from build123d import *

# Parameters (mm, degrees)
PAD001_DEPTH    = 28.5
SKETCH002_R     = 14.25
POCKET_DEPTH    = 18.5
SKETCH003_R     = 1.375
POCKET001_DEPTH = 10
CHAMFER_SIZE    = 1
SKETCH004_W     = 10.5
SKETCH004_H     = 4
POCKET002_DEPTH = 10
SKETCH008_R     = 3
POCKET004_DEPTH = 5
SKETCH009_R     = 1.75
POCKET005_DEPTH = 5
CHAMFER004_SIZE = 0.5
SKETCH012_R     = 1.375
POCKET008_DEPTH = 8
SKETCH013_R     = 1.375
POCKET009_DEPTH = 8
CHAMFER005_SIZE = 1


with BuildPart() as motorbracketgroovemirrored001:
    # Sketch001 → Pad001 (new body)
    with BuildSketch(Plane.YZ):
        with BuildLine():
            ThreePointArc((2.474858, 19.974889), (-1.339402, 20.733574), (-3.5, 17.5))
            Line((-3.5, 17.5), (-3.5, -17.5))
            ThreePointArc((-3.5, -17.5), (-1.339402, -20.733574), (2.474858, -19.974889))
            Line((4.5, -17.949747), (2.474858, -19.974889))
            Line((4.5, 17.949747), (4.5, -17.949747))
            Line((4.5, 17.949747), (2.474858, 19.974889))
        make_face()
    extrude(amount=PAD001_DEPTH)

    # Sketch002 → Pocket (cut)
    with BuildSketch(Plane.YZ.offset(28.5)):
        Circle(SKETCH002_R)
    extrude(amount=-POCKET_DEPTH, mode=Mode.SUBTRACT)

    # Sketch003 → Pocket001 (cut)
    with BuildSketch(Plane.YZ.offset(28.5)):
        with Locations((0, 17.5)):
            Circle(SKETCH003_R)
    pocket001 = extrude(amount=-POCKET001_DEPTH, mode=Mode.SUBTRACT)

    # Mirrored: Pocket001 across Sketch003 H_Axis
    add(pocket001.mirror(Plane(origin=(28.5, 0, 0), x_dir=(1, 0, 0), z_dir=(0, 0, 1))), mode=Mode.SUBTRACT)

    # Chamfer
    chamfer_edges = [motorbracketgroovemirrored001.edges().sort_by_distance(p)[0] for p in [
        (28.5, -1.375, 17.5),
        (28.5, -1.375, -17.5),
    ]]
    chamfer(chamfer_edges, length=CHAMFER_SIZE)

    # Sketch004 → Pocket002 (cut)
    with BuildSketch(Plane(origin=(0, 4.5, 0), x_dir=(-1, 0, 0), z_dir=(0, 1, 0))):
        with Locations((-5.25, 20)):
            Rectangle(SKETCH004_W, SKETCH004_H)
    pocket002 = extrude(amount=-POCKET002_DEPTH, mode=Mode.SUBTRACT)

    # Mirrored001: Pocket002 across Sketch004 H_Axis
    add(pocket002.mirror(Plane(origin=(0, 4.5, 0), x_dir=(0, 1, 0), z_dir=(0, 0, 1))), mode=Mode.SUBTRACT)


with BuildPart() as motorbracketscrewchamfer005_final:
    # Part__Mirroring: instance of MotorBracketGrooveMirrored001
    add(motorbracketgroovemirrored001.part.mirror(Plane(origin=(0, 0, 0), x_dir=(0, -1, 0), z_dir=(1, 0, 0))))

    # Fusion001: union MotorBracketGrooveMirrored001
    add(motorbracketgroovemirrored001.part)

    # Sketch008 → Pocket004 (cut)
    with BuildSketch(Plane.XZ.offset(3.5)):
        Circle(SKETCH008_R)
    extrude(amount=-POCKET004_DEPTH, mode=Mode.SUBTRACT)

    # Sketch009 → Pocket005 (cut)
    with BuildSketch(Plane.XZ.offset(-1.5)):
        Circle(SKETCH009_R)
    extrude(amount=-POCKET005_DEPTH, mode=Mode.SUBTRACT)

    # Chamfer004
    chamfer004_edges = [motorbracketscrewchamfer005_final.edges().sort_by_distance(p)[0] for p in [
        (10, 4.5, 0),
        (0, 4.5, 1.75),
        (-10, 4.5, 0),
        (-28.5, 4.5, -15.735282),
        (-28.5, 4.5, 15.735282),
        (28.5, 4.5, -15.735282),
        (28.5, 4.5, 15.735282),
    ]]
    chamfer(chamfer004_edges, length=CHAMFER004_SIZE)

    # Sketch012 → Pocket008 (cut)
    with BuildSketch(Plane.XY.offset(18)):
        with Locations((0, 0.5)):
            Circle(SKETCH012_R)
    extrude(amount=-POCKET008_DEPTH, mode=Mode.SUBTRACT)

    # Sketch013 → Pocket009 (cut)
    with BuildSketch(Plane(origin=(0, 0, -18), x_dir=(1, 0, 0), z_dir=(0, 0, -1))):
        with Locations((0, -0.5)):
            Circle(SKETCH013_R)
    extrude(amount=-POCKET009_DEPTH, mode=Mode.SUBTRACT)

    # Chamfer005
    chamfer005_edges = [motorbracketscrewchamfer005_final.edges().sort_by_distance(p)[0] for p in [
        (-1.375, 0.5, -18),
        (-1.375, 0.5, 18),
    ]]
    chamfer(chamfer005_edges, length=CHAMFER005_SIZE)


solid = motorbracketscrewchamfer005_final.part
Verification items for the finished model (mm, model axes). A direction names the side the tool comes from. Coordinates: 2 decimals unless noted, no trailing zeros. Loops run counter-clockwise (first coordinate to the right, second up) from the corner with the lowest first, then second, coordinate; pieces in that order, holes last. Notation, with made-up numbers: (-18, -35.5) -> (-1, -35.5) arc R30 ccw to (-1, -7.5) -> close; hole circle Ø1 at (-5, 8). An arc over 180 degrees is marked (long way). Answer as a JSON object with one key per item and string values. Group by question number.
Item 1: Scan lines: probe 1 along Z at (x, y) = (-21.5, 0) (3 decimals); probe 2 along Y at (x, z) = (0, 11.5) (3 decimals); probe 3 along Z at (x, y) = (19, 0.75). Record each from-to range of solid material in increasing order.
Item 2: Mould release check, pull along X, two halves, no side actions. Record for faces 1 (the flat face through (0, 4.5, -4)), 2 (the flat face through (-10.5, 1, 19)), 3 (the flat face through (28.5, 0.2, 14.9)): +X half, -X half, draft (parallel to the pull), parting line (faces both ways), or undercut.
Item 3: Tool access check on faces 4 (the cylindrical face through (-23.063, -0.179, -18.863)), 5 (the flat face through (18.5, 0, -18)), 6 (the flat face through (2.5, -0.3, 18)), 7 (the flat face through (0, 1.5, -2)). Record the directions out of +Z, -Z, +X, -X, +Y, -Y that give a thin tool (end or side, any length) a straight path to the whole face; none if there is none.
Item 4: Depth check by flat-ended pin: pin 1 (2 mm diameter, centred on x = 0, y = 0.5, fed in from +Z); pin 2 (0.8 mm diameter, centred on x = -0.5, y = 0.5, fed in from -Z); pin 3 (1 mm diameter, centred on x = -18.5, y = 2.5, fed in from -Z). Enter the tip coordinate at first touch or a pass-through.
Item 5: Sectioned sample at C-C on x = -23.5. Record the boundary of the cut face in (y, z) (3 decimals), plus the area to 3 significant figures.
Item 6: Sectioned sample at A-A on z = 0. Record the boundary of the cut face in (x, y).
Evaluation:
{
 "1": {"probe 1": "z = -21 to -18.875, -16.125 to -14.25, 14.25 to 16.125, 18.875 to 21", "probe 2": "y = -3.5 to -0.875, 1.875 to 4.5", "probe 3": "z = -20.92 to -18.65, -16.35 to -14.23, 14.23 to 16.35, 18.65 to 20.92"},
 "2": {"face 1": "draft", "face 2": "undercut", "face 3": "+X half"},
 "3": {"face 4": "-X", "face 5": "+X", "face 6": "+Z, +Y, -Y", "face 7": "-Y"},
 "4": {"pin 1": "stops at z = 10", "pin 2": "stops at z = -10", "pin 3": "stops at z = -20.37"},
 "5": {"outline": "(-3.5, -17.5) arc R3.5 ccw to (2.475, -19.975) -> (4.5, -17.95) -> (4.5, -13.521) arc R14.25 cw to (-3.5, -13.813) -> close; (-3.5, 13.813) arc R14.25 cw to (4.5, 13.521) -> (4.5, 17.95) -> (2.475, 19.975) arc R3.5 ccw to (-3.5, 17.5) -> close; hole circle Ø2.75 at (0, -17.5); hole circle Ø2.75 at (0, 17.5)", "area": "84.2 mm²"},
 "6": {"outline": "(-10, -3.5) -> (-3, -3.5) -> (-3, 1.5) -> (-1.75, 1.5) -> (-1.75, 4) -> (-2.25, 4.5) -> (-9.5, 4.5) -> (-10, 4) -> close; (1.75, 1.5) -> (3, 1.5) -> (3, -3.5) -> (10, -3.5) -> (10, 4) -> (9.5, 4.5) -> (2.25, 4.5) -> (1.75, 4) -> close"}
}
